Input: part model. Units: mm. Frame: model coordinates. Round coordinates to 2 decimals unless told otherwise and drop trailing zeros. Loops run counter-clockwise (first coordinate to the right, second up) from the corner with the lowest first, then second, coordinate; pieces in that order, holes last. Notation, with made-up numbers: (21, 51.5) -> (61, 51.5) arc R28 cw to (61, 83.5) -> close; hole circle Ø5 at (-24, 25). An arc over 180 degrees is marked (long way). Answer as a JSON object with one key per item and string values. Group by question number.
Item 1: Section query C-C on x = 50. Return loops of the section in (y, z), and give its area (3 significant figures).
Item 2: Section query B-B on z = 28. Return loops of the section in (x, y).
Item 3: Pin query (flat end, axial travel): pin 1 (2.5 mm diameter, centred on y = 34.5, z = -1.5, fed in from -X); pin 2 (4 mm diameter, centred on y = 38, z = 7.5, fed in from -X); pin 3 (4 mm diameter, centred on y = 64, z = 44, fed in from -X); pin 4 (22 mm diameter, centred on x = 77.5, y = 61.5, fed in from +Z). Return the tip coordinate at first contact, or that it passes through.
Item 4: Section query A-A on y = 47.5. Return loops of the section in (x, z), and give its area (3 significant figures).
Item 5: Section query D-D on x = 106.5. Return loops of the section in (y, z).
Item 6: Material intervals for line 1 (Y direction, x = 32, z = 15); line 2 (X direction, y = 59.5, z = 41.5); line 3 (X direction, y = 46, z = 4), sorted ascending. Write a range as [from, to].
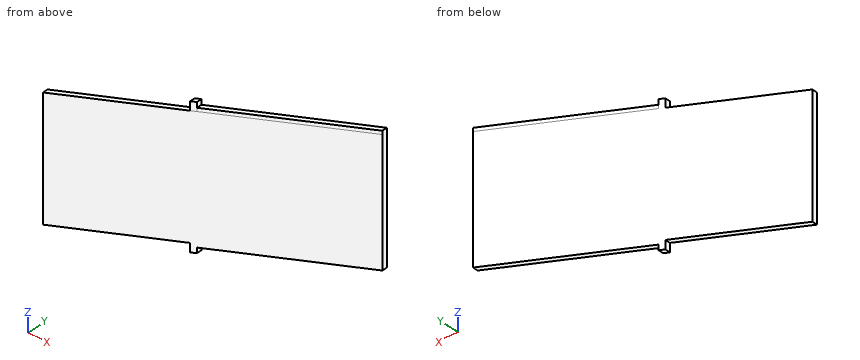
Autodesk Inventor part; units mm, degrees
ref_plane "YZ Plane" through (0, 0, 0) normal (1, 0, 0) x (0, 1, 0)
ref_plane "XZ Plane" through (0, 0, 0) normal (0, 1, 0) x (-1, 0, 0)
ref_plane "XY Plane" through (0, 0, 0) normal (0, 0, 1) x (1, 0, 0)
sketch "Sketch6" plane through (0, 0, 0) normal (0, 0, 1) x (1, 0, 0)
  line L0 (0, 0) -> (0, 3)
  line L1 (0, 3) -> (129.9038, 78)
  line L2 (129.9038, 78) -> (129.9038, 75)
  line L3 (129.9038, 75) -> (0, 0)
  dimension "d18" = 3
  dimension "d19" = 150
  dimension "d20" = 120
  dimension "d21" = 3
extrude "Extrusion6" add sketch "Sketch6" along normal blind 70
sketch "Sketch8" plane through (0, 0, 70) normal (0, 0, 1) x (1, 0, 0)
  line L0 (56.2917, 35.5) -> (56.2917, 32.5)
  line L1 (129.9038, 78) -> (0, 3)
  line L2 (56.2917, 32.5) -> (58.8897, 34)
  line L3 (129.9038, 75) -> (0, 0)
  line L4 (58.8897, 34) -> (58.8897, 37)
  line L5 (0, 3) -> (129.9038, 78)
  line L6 (56.2917, 35.5) -> (58.8897, 37)
  line L7 (56.2917, 35.5) -> (56.2917, 32.5)
  dimension "d27" = 3
extrude "Extrusion8" add sketch "Sketch8" along normal blind 5
sketch "Sketch9" plane through (0, 0, 70) normal (0, 0, 1) x (1, 0, 0)
  line L0 (58.8897, 37) -> (58.8897, 34)
  line L1 (58.8897, 34) -> (129.9038, 75)
  line L2 (129.9038, 75) -> (129.9038, 78)
  line L3 (129.9038, 78) -> (58.8897, 37)
  point P0 (0, 0)
extrude "Extrusion9" add sketch "Sketch9" along normal blind 2
sketch "Sketch10" plane through (0, 0, 0) normal (0, 0, -1) x (-1, 0, 0)
  line L0 (0, 3) -> (-129.9038, 78)
  line L1 (-129.9038, 75) -> (0, 0)
  line L2 (0, 3) -> (-56.2917, 35.5)
  line L3 (-56.2917, 35.5) -> (-58.8897, 37)
  line L4 (-58.8897, 37) -> (-58.8897, 34)
  line L5 (0, 0) -> (-56.2917, 32.5)
  line L6 (-58.8897, 34) -> (-56.2917, 32.5)
  line L7 (-56.2917, 35.5) -> (-56.2917, 32.5)
  line L8 (-56.2917, 32.5) -> (-56.2917, 35.5)
  point P0 (-64.9519, 37.5)
  dimension "d32" = 65
  dimension "d33" = 3
extrude "Extrusion10" add sketch "Sketch10" along normal blind 5
sketch "Sketch11" plane through (0, 0, 0) normal (0, 0, -1) x (-1, 0, 0)
  line L0 (-58.8897, 34) -> (-58.8897, 37)
  line L1 (0, 3) -> (-129.9038, 78)
  line L2 (-129.9038, 78) -> (-129.9038, 75)
  line L3 (-129.9038, 75) -> (0, 0)
extrude "Extrusion11" add sketch "Sketch11" along normal blind 2
properties part number "Zonnepaneel V5.0 print Versie"
Solved:
{
 "1": {"outline": "(28.87, 0) -> (31.87, 0) -> (31.87, 70) -> (28.87, 70) -> close", "area": "210 mm²"},
 "2": {"outline": "(0, 0) -> (129.9, 75) -> (129.9, 78) -> (0, 3) -> close"},
 "3": {"pin 1": "x = 56.29", "pin 2": "x = 57.16", "pin 3": "x = 102.19", "pin 4": "through"},
 "4": {"outline": "(77.08, -2) -> (82.27, -2) -> (82.27, 72) -> (77.08, 72) -> close", "area": "385 mm²"},
 "5": {"outline": "(61.49, -2) -> (64.49, -2) -> (64.49, 72) -> (61.49, 72) -> close"},
 "6": {"line 1": "[18.48, 21.48]", "line 2": "[97.86, 103.06]", "line 3": "[74.48, 79.67]"}
}
